The figure shows three views and two pictorial views of one solid part (mm, origin at its lowest corner). Answer the questions. Round coordinates to 2 decimals unless told otherwise and drop trailing zeros. Order: outer loops, then holes, each group sorted by start corner. A loop starts at its lowest first (then second) coordinate and runs counter-clockwise, first axis right, second up. Notation, with made-up numbers: (40, -28.5) -> (73, -28.5) arc R5 cw to (73, -24.5) -> close; hole circle Ø10 at (-7, 41.25). An arc over 180 degrees is marked (long way). Answer as a JSON object with one key per item and string values. Group by question number.
Item 1: Consider probe 1 along X at (y, z) = (3.75, 0.2) (1 decimal); probe 2 along X at (y, z) = (8, 0.35); probe 3 along Y at (x, z) = (22.75, 0.1) (1 decimal). Determine where each line is inside the solid, lowest interval first. Write a range as from..to.
Item 2: Section B-B, the plane y = 4.75 is taken. Write down the section's boundary in (x, z).
Item 3: Section C-C, the plane x = 2.75 is taken. Write down the section's boundary in (y, z) (1 decimal).
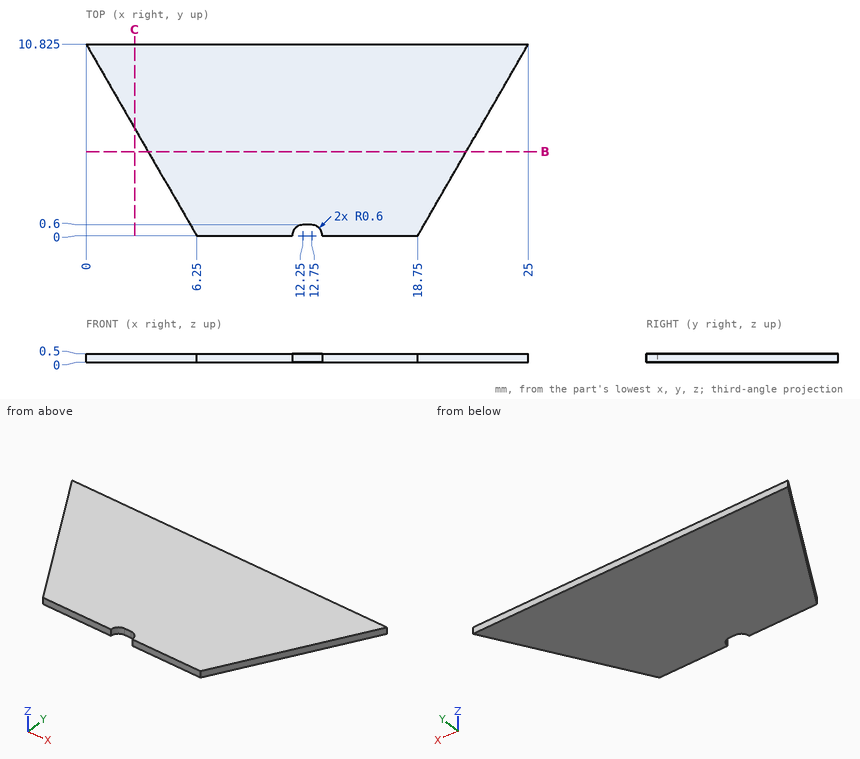
Values found:
{
 "1": {"probe 1": "4.1..20.9", "probe 2": "1.63..23.37", "probe 3": "6.9..10.8"},
 "2": {"outline": "(3.51, 0) -> (21.49, 0) -> (21.49, 0.5) -> (3.51, 0.5) -> close"},
 "3": {"outline": "(6.1, 0) -> (10.8, 0) -> (10.8, 0.5) -> (6.1, 0.5) -> close"}
}
